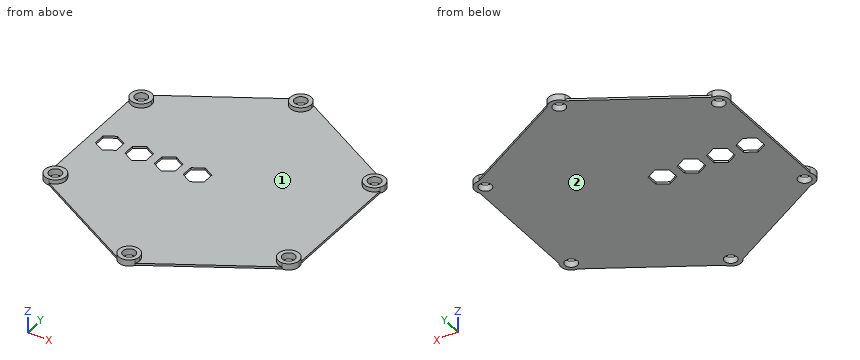
from build123d import *

# Parameters (mm, degrees)
F1_DEPTH = 1
F0_R     = 3
F2_DEPTH = 3


with BuildPart() as f1:
    # F0 (on Top) → F1 (new body)
    with BuildSketch(Plane.XY):
        with BuildLine():
            Line((60, -29.5747704777), (60, 29.574769431))
            ThreePointArc((60, 29.574769431), (51.3994928411, 29.6755110105), (55.6125027826, 37.1741388509))
            Line((55.6125027826, 37.1741388509), (4.3874976328, 66.7489093634))
            ThreePointArc((4.3874976328, 66.7489093634), (4.844454983, 65.5884611093), (5, 64.351021851))
            ThreePointArc((5, 64.351021851), (-1.2374392583, 59.506566868), (-4.3874976328, 66.7489093634))
            Line((-4.3874976328, 66.7489093634), (-55.6125023294, 37.1741391126))
            ThreePointArc((-55.6125023294, 37.1741391126), (-52.1529183527, 35.6693921891), (-50.7296198931, 32.1755109531))
            ThreePointArc((-50.7296198931, 32.1755109531), (-54.37904604, 27.3613702959), (-60, 29.5747699543))
            Line((-60, 29.5747699543), (-60, -29.5747699543))
            ThreePointArc((-60, -29.5747699543), (-54.3790460573, -27.3613707384), (-50.7296201258, -32.1755113351))
            ThreePointArc((-50.7296201258, -32.1755113351), (-52.152918285, -35.6693922636), (-55.6125017026, -37.1741394744))
            Line((-55.6125017026, -37.1741394744), (-4.3874984862, -66.7489088707))
            ThreePointArc((-4.3874984862, -66.7489088707), (-1.237438708, -59.5065674728), (4.9999998449, -64.351022636))
            ThreePointArc((4.9999998449, -64.351022636), (4.8444549712, -65.5884613333), (4.387498033, -66.7489091323))
            Line((4.387498033, -66.7489091323), (55.6125012494, -37.1741397361))
            ThreePointArc((55.6125012494, -37.1741397361), (51.3994931648, -29.6755112347), (60, -29.5747704777))
        make_face()
        Polygon((-8.3002293408, -5.8508351856), (-13.3002293408, -2.9640838396), (-13.3002293408, 2.8094188523), (-8.3002293408, 5.6961701982), (-3.3002293408, 2.8094188523), (-3.3002293408, -2.9640838396), align=None, mode=Mode.SUBTRACT)
        Polygon((-50.3002293408, 5.7735026919), (-45.3002293408, 2.8867513459), (-45.3002293408, -2.8867513459), (-50.3002293408, -5.7735026919), (-55.3002293408, -2.8867513459), (-55.3002293408, 2.8867513459), align=None, mode=Mode.SUBTRACT)
        Polygon((-36.3002293408, -5.6435510621), (-41.3002293408, -2.7567997162), (-41.3002293408, 3.0167029757), (-36.3002293408, 5.9034543217), (-31.3002293408, 3.0167029757), (-31.3002293408, -2.7567997162), align=None, mode=Mode.SUBTRACT)
        Polygon((-22.3002293408, -5.5399089458), (-27.3002293408, -2.6531575999), (-27.3002293408, 3.120345092), (-22.3002293408, 6.007096438), (-17.3002293408, 3.120345092), (-17.3002293408, -2.6531575999), align=None, mode=Mode.SUBTRACT)
    extrude(amount=F1_DEPTH)

    # F0 (on Top) → F2 (join)
    with BuildSketch(Plane.XY):
        with BuildLine():
            ThreePointArc((-50.7296198931, 32.1755109531), (-52.1529183527, 35.6693921891), (-55.6125023294, 37.1741391126))
            ThreePointArc((-55.6125023294, 37.1741391126), (-60.0597469512, 34.6755108854), (-60, 29.5747699543))
            ThreePointArc((-60, 29.5747699543), (-54.37904604, 27.3613702959), (-50.7296198931, 32.1755109531))
        make_face()
        with Locations((-55.7296198931, 32.1755109531)):
            Circle(F0_R, mode=Mode.SUBTRACT)
        with BuildLine():
            ThreePointArc((5, 64.351021851), (4.844454983, 65.5884611093), (4.3874976328, 66.7489093634))
            ThreePointArc((4.3874976328, 66.7489093634), (0, 69.351021851), (-4.3874976328, 66.7489093634))
            ThreePointArc((-4.3874976328, 66.7489093634), (-1.2374392583, 59.506566868), (5, 64.351021851))
        make_face()
        with Locations((0, 64.351021851)):
            Circle(F0_R, mode=Mode.SUBTRACT)
        with BuildLine():
            ThreePointArc((55.6125027826, 37.1741388509), (51.3994928411, 29.6755110105), (60, 29.574769431))
            ThreePointArc((60, 29.574769431), (60.5437606651, 30.8249366878), (60.7296200482, 32.1755106845))
            ThreePointArc((60.7296200482, 32.1755106845), (59.2235013908, 35.7522121207), (55.6125027826, 37.1741388509))
        make_face()
        with Locations((55.7296200482, 32.1755106845)):
            Circle(F0_R, mode=Mode.SUBTRACT)
        with BuildLine():
            ThreePointArc((60.7296199707, -32.1755116038), (60.5437606077, -30.8249376789), (60, -29.5747704777))
            ThreePointArc((60, -29.5747704777), (51.3994931648, -29.6755112347), (55.6125012494, -37.1741397361))
            ThreePointArc((55.6125012494, -37.1741397361), (59.2235007925, -35.7522135487), (60.7296199707, -32.1755116038))
        make_face()
        with Locations((55.7296199707, -32.1755116038)):
            Circle(F0_R, mode=Mode.SUBTRACT)
        with BuildLine():
            ThreePointArc((-4.3874984862, -66.7489088707), (-3.042e-07, -69.351022636), (4.387498033, -66.7489091323))
            ThreePointArc((4.387498033, -66.7489091323), (4.8444549712, -65.5884613333), (4.9999998449, -64.351022636))
            ThreePointArc((4.9999998449, -64.351022636), (-1.237438708, -59.5065674728), (-4.3874984862, -66.7489088707))
        make_face()
        with Locations((-1.551e-07, -64.351022636)):
            Circle(F0_R, mode=Mode.SUBTRACT)
        with BuildLine():
            ThreePointArc((-60, -29.5747699543), (-60.0597470807, -34.6755114459), (-55.6125017026, -37.1741394744))
            ThreePointArc((-55.6125017026, -37.1741394744), (-52.152918285, -35.6693922636), (-50.7296201258, -32.1755113351))
            ThreePointArc((-50.7296201258, -32.1755113351), (-54.3790460573, -27.3613707384), (-60, -29.5747699543))
        make_face()
        with Locations((-55.7296201258, -32.1755113351)):
            Circle(F0_R, mode=Mode.SUBTRACT)
    extrude(amount=F2_DEPTH)


solid = f1.part
Source: CAD feature listing. Evaluate the final solid. Frame: model axes, mm. Face numbers are marked on the shaded views. Round coordinates to 2 decimals unless told otherwise and drop trailing zeros. Loops run counter-clockwise (first coordinate to the right, second up) from the corner with the lowest first, then second, coordinate; pieces in that order, holes last.
Q1. Section A-A, the plane z = 2.3. State how many separate pieces and enclosed holes the cut face has, plus the area to 3 significant figures.
Q2. Section B-B, the plane x = 0. Return loops of the section in (y, z).
Q3. Ray query, line 1 (X direction, y = 32, z = 2.4); line 2 (Y direction, x = -1, z = 2.85); line 3 (X direction, y = -20.5, z = 0.3). Return the intervals inside material, ascending.
Q4. Mould query, pull axis X, two halves, no side actions, for the marked faces 1 and 2. Classes: pulls with the +X half, pulls with the -X half, needs draft (parallel to the pull), parting line crosses it, or undercut.
Q5. Section C-C, the plane x = 33. Return loops of the section in (y, z).
Q6. First-contact query: P1, Ø0.8, axis at y = 14.5, z = 0.5, coming from the +X side; P2, Ø10, axis at x = 12.5, y = -6, coming from the +Z side; P3, Ø5.5, axis at x = -55.73, y = -32.18, coming from the -Z side; P4, Ø1.1, axis at y = 0.5, z = 0.5, coming from the -X side. Flat tips, straight axial feed; report the tip coordinate or a pass-through.
Q7. Section D-D, the plane y = -39.5. Return loops of the section in (x, z), plus the area to 3 significant figures.
Solutions:
1. separate pieces: 6
1. enclosed holes: 6
1. area: 302 mm2
2. outline: (-69.35, 0) - (-67.35, 0) - (-67.35, 3) - (-69.35, 3) - close; (-61.35, 0) - (61.35, 0) - (61.35, 3) - (59.35, 3) - (59.35, 1) - (-59.35, 1) - (-59.35, 3) - (-61.35, 3) - close; (67.35, 0) - (69.35, 0) - (69.35, 3) - (67.35, 3) - close
3. line 1: x = -60.73 to -58.72, -52.73 to -50.73, 50.73 to 52.73, 58.72 to 60.73
3. line 2: y = -69.25 to -67.18, -61.52 to -59.45, 59.45 to 61.52, 67.18 to 69.25
3. line 3: x = -60 to 60
4. face 1: undercut
4. face 2: needs draft
5. outline: (-50.23, 0) - (50.23, 0) - (50.23, 1) - (-50.23, 1) - close
6. P1: stops at x = 60
6. P2: stops at z = 1
6. P3: passes through
6. P4: stops at x = -60
7. outline: (-51.58, 0) - (51.58, 0) - (51.58, 1) - (-51.58, 1) - close
7. area: 103 mm2
